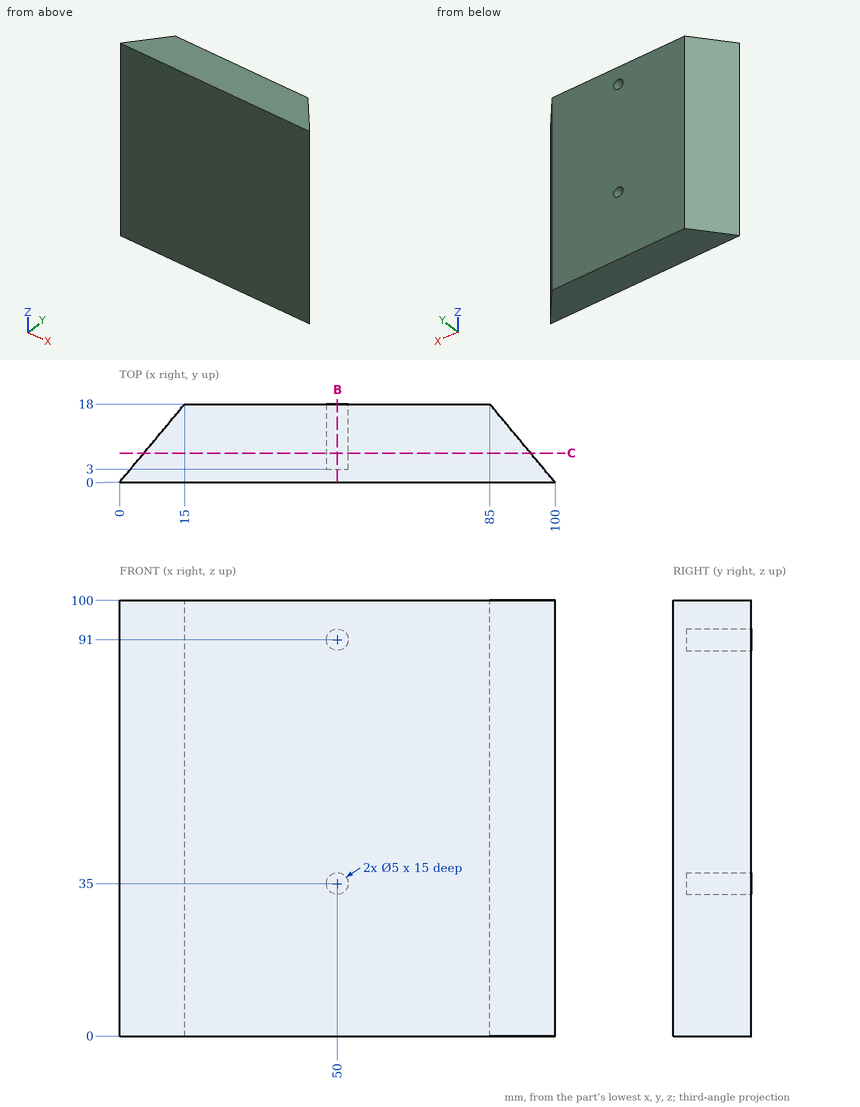
Job drawing, mm, ordinate dimensions from the low corner. One solid piece. Round coordinates to 2 decimals unless told otherwise and drop trailing zeros. Loops run counter-clockwise (first coordinate to the right, second up) from the corner with the lowest first, then second, coordinate; pieces in that order, holes last.
Item 1: Drill centre lines: line 1 (Z direction, x = 50, y = 8); line 2 (X direction, y = 9.5, z = 91); line 3 (X direction, y = 10.75, z = 91). Where is each one in solid material? Low to high.
Item 2: Drop flat-ended pins along their axis: P1, Ø1.5, axis at y = 5.5, z = 15.5, coming from the -X side; P2, Ø1.5, axis at y = 3, z = 17.5, coming from the -X side (3 decimals); P3, Ø4, axis at x = 50, z = 91, coming from the +Y side. Give the stop position or say it passes through.
Item 3: Cut at B-B, the plane x = 50. Give the cut face in (y, z), then the cut area to 3 significant figures.
Item 4: Cut at C-C, the plane y = 6.75. Give the cut face in (x, z) (3 decimals), then the cut area to 3 significant figures.
A:
1. line 1: z = 0 to 32.5, 37.5 to 88.5, 93.5 to 100
1. line 2: x = 7.92 to 47.5, 52.5 to 92.08
1. line 3: x = 8.96 to 47.5, 52.5 to 91.04
2. P1: stops at x = 3.96
2. P2: stops at x = 1.875
2. P3: stops at y = 3
3. outline: (0, 0) - (18, 0) - (18, 32.5) - (3, 32.5) - (3, 37.5) - (18, 37.5) - (18, 88.5) - (3, 88.5) - (3, 93.5) - (18, 93.5) - (18, 100) - (0, 100) - close
3. area: 1,650 mm2
4. outline: (5.625, 0) - (94.375, 0) - (94.375, 100) - (5.625, 100) - close; hole circle Ø5 at (50, 35); hole circle Ø5 at (50, 91)
4. area: 8,840 mm2
